from build123d import *

# Parameters (mm, degrees)
SKETCH1_R           = 2.1
BOSS_EXTRUDE1_DEPTH = 2


with BuildPart() as part:
    # Sketch1 → Boss-Extrude1 (new body)
    with BuildSketch(Plane.XY):
        with BuildLine():
            ThreePointArc((23.881885124, -2.44114481), (24.246083691, -3.99705075), (25.842354675, -3.923546751))
            ThreePointArc((25.842354675, -3.923546751), (39.627475181, 2.225248194), (54.35720616, -1.072061603))
            ThreePointArc((54.35720616, -1.072061603), (55.945448574, -0.81769615), (55.968200147, 0.79062537))
            ThreePointArc((55.968200147, 0.79062537), (26.805089731, 15.449219208), (-3.569399351, 3.501340925))
            ThreePointArc((-3.569399351, 3.501340925), (-3.398562383, -3.667393315), (3.762428977, -3.293042391))
            ThreePointArc((3.762428977, -3.293042391), (9.440329247, 1.908120602), (16.118141008, 5.741849601))
            ThreePointArc((16.118141008, 5.741849601), (22.86761221, 4.371031998), (23.881885124, -2.44114481))
        make_face()
        Circle(SKETCH1_R, mode=Mode.SUBTRACT)
    extrude(amount=BOSS_EXTRUDE1_DEPTH)


solid = part.part
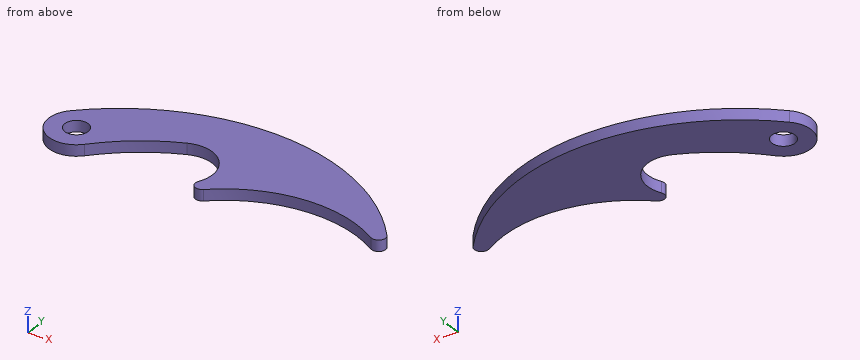
For this review, take the finished solid that the model builds, in its own axes (mm). Coordinates: 2 decimals unless noted, no trailing zeros. Order: outer loops, then holes, each group sorted by start corner. A loop starts at its lowest first (then second) coordinate and runs counter-clockwise, first axis right, second up. Notation, with made-up numbers: (-35, 26.25) - (12, 26.25) arc R15 ccw to (12, 43.25) - close; hole circle Ø6 at (86, -7.5). An arc over 180 degrees is marked (long way). Answer as CSV lines item,"result". Start each with the question number.
1) Add section C-C (z = 0.3). State the section outline as (x, y) points, then the cut area to 3 significant figures.
2) Add section D-D (x = 42). State the section outline as (y, z) points.
3) Insertion check: P1, Ø4, axis at x = 0, y = 0, coming from the -Z side; P2, Ø1, axis at y = 12.5, z = 1, coming from the +X side. Each pin has a flat end and moves straight along its axis. Give the tip position at first contact, or say it passes through.
4) Add section A-A (y = 0). State the section outline as (x, z) points.
5) Add section B-B (x = 0). State the section outline as (y, z) points.
6) To check wall thickness, follow line 1 along Y through (x, z) = (0, 1); line 2 along Y through (x, z) = (1, 0.4); line 3 along Y through (x, z) = (53.5, 1). State the ranges of each line that lie inside material, in increasing order. Write a range as [from, to].
Result:
1,outline,"(-3.57, 3.5) arc R5 ccw (long way) to (3.76, -3.29) arc R35 cw to (16.12, 5.74) arc R6 cw to (23.88, -2.44) arc R1.25 ccw to (25.84, -3.92) arc R24 cw to (54.36, -1.07) arc R1.25 ccw to (55.97, 0.79) arc R40 ccw to start; hole circle Ø4.2 at (0, 0)"
1,area,"623 mm^2"
2,outline,"(2.34, 0) - (11.69, 0) - (11.69, 2) - (2.34, 2) - close"
3,P1,"through"
3,P2,"x = 41.33"
4,outline,"(-5, 0) - (-2.1, 0) - (-2.1, 2) - (-5, 2) - close; (2.1, 0) - (7.06, 0) - (7.06, 2) - (2.1, 2) - close; (24.51, 0) - (31.67, 0) - (31.67, 2) - (24.51, 2) - close; (52.36, 0) - (56.25, 0) - (56.25, 2) - (52.36, 2) - close"
5,outline,"(-5, 0) - (-2.1, 0) - (-2.1, 2) - (-5, 2) - close; (2.1, 0) - (6.73, 0) - (6.73, 2) - (2.1, 2) - close"
6,line 1,"[-5, -2.1], [2.1, 6.73]"
6,line 2,"[-4.9, -1.85], [1.85, 7.5]"
6,line 3,"[-0.58, 3.54]"
